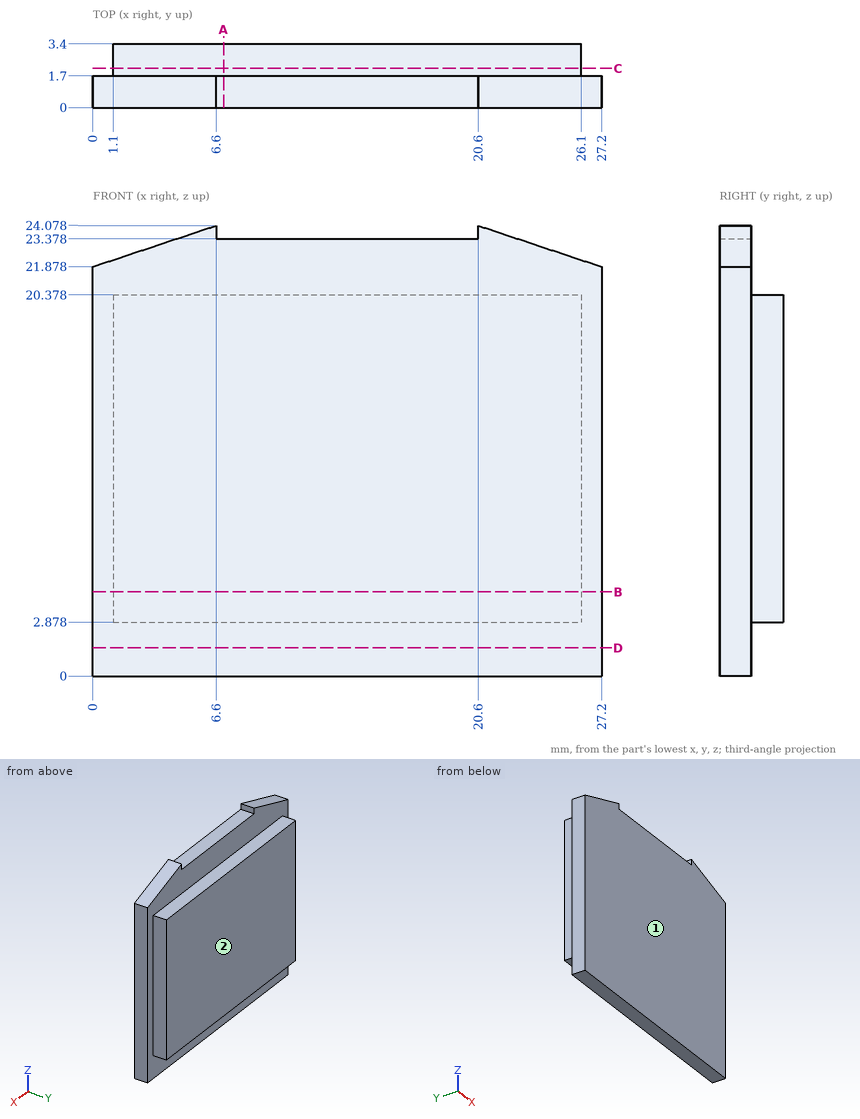
The figure shows three views and two pictorial views of one solid part (mm, origin at its lowest corner). Answer the questions. Round coordinates to 2 decimals unless told otherwise and drop trailing zeros. Order: outer loops, then holes, each group sorted by start corner. A loop starts at its lowest first (then second) coordinate and runs counter-clockwise, first axis right, second up. Notation, with made-up numbers: M -24.75,14.25 L 1.25,14.25 A4 cw 1.25,21.25 Z; hole C 77,-3.75 d9. An arc over 180 degrees is marked long. Put each result on its own line as item: value. Start each with the question number.
Q1. Section B-B, the plane z = 4.5 is taken. Write down the section's boundary in (x, y).
Q2. Straight lines are drawn through the part: L1, parallel to Z at x = 14.25, y = 3.2; L2, parallel to X at y = 2, z = 11.5; L3, parallel to Z at x = 11.75, y = 0.95. For each, find the intervals that lie inside material, in ascending order. Write a range as [from, to].
Q3. Section D-D, the plane z = 1.5 is taken. Write down the section's boundary in (x, y), and give its area (3 significant figures).
Q4. Section A-A, the plane x = 7 is taken. Write down the section's boundary in (y, z), and give its area (3 significant figures).
Q5. For a pull along Y with two mould halves and no side action, classify the marked faces 1 and 2 as pulls with the +Y half, pulls with the -Y half, needs draft (parallel to the pull), parting line crosses it, or undercut.
Q6. Flat-ended cylindrical pins translate along their axes: pin 1 (1.5 mm diameter, centred on x = 4.5, y = 0.5, fed in from +Z); pin 2 (0.8 mm diameter, centred on x = 12.5, y = 2.5, fed in from -Z); pin 3 (0.8 mm diameter, centred on y = 3, z = 8, fed in from -X). Find the tip coordinate at first contact, or state that the pin passes through.
Q7. Section C-C, the plane y = 2.1 is taken. Write down the section's boundary in (x, z).
Findings below:
1. outline: M 0,0 L 27.2,0 L 27.2,1.7 L 26.1,1.7 L 26.1,3.4 L 1.1,3.4 L 1.1,1.7 L 0,1.7 Z
2. L1: z = [2.88, 20.38]
2. L2: x = [1.1, 26.1]
2. L3: z = [0, 23.38]
3. outline: M 0,0 L 27.2,0 L 27.2,1.7 L 0,1.7 Z
3. area: 46.2 mm^2
4. outline: M 0,0 L 1.7,0 L 1.7,2.88 L 3.4,2.88 L 3.4,20.38 L 1.7,20.38 L 1.7,23.38 L 0,23.38 Z
4. area: 69.5 mm^2
5. face 1: pulls with the -Y half
5. face 2: pulls with the +Y half
6. pin 1: stops at z = 23.63
6. pin 2: stops at z = 2.88
6. pin 3: stops at x = 1.1
7. outline: M 1.1,2.88 L 26.1,2.88 L 26.1,20.38 L 1.1,20.38 Z
